Here's the drawing with two shaded views (mm, measured from the low corner). I have some questions. A direction names the side the tool comes from. Coordinates: 2 decimals unless noted, no trailing zeros. Loops run counter-clockwise (first coordinate to the right, second up) from the corner with the lowest first, then second, coordinate; pieces in that order, holes last. Notation, with made-up numbers: (86, 72) - (111, 72) arc R21 ccw to (111, 109) - close; hole circle Ø7 at (89, -12). An arc over 180 degrees is marked (long way). Use a Markdown table: item, result.
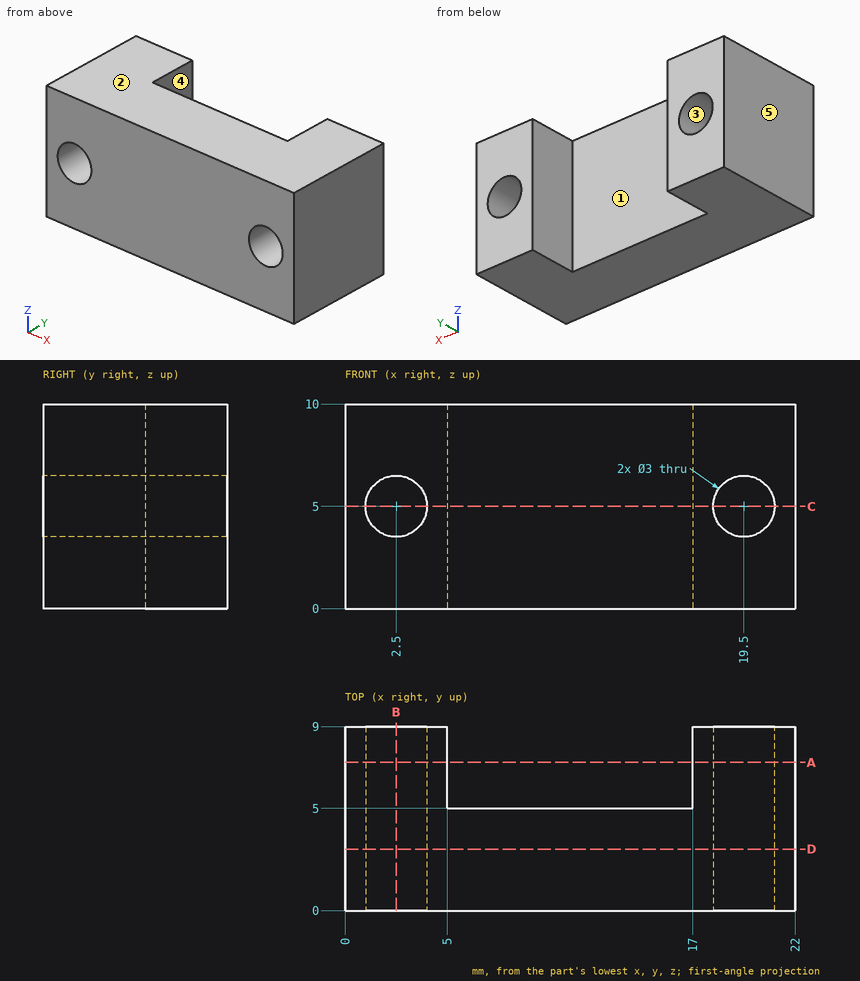
Q1. Please list where these lines run through material, in increasing order: L1, parallel to X at y = 2.5, z = 5; L2, parallel to Z at x = 19.5, y = 5; L3, parallel to X at y = 1.75, z = 6.25. Write a range as from..to.
Check values:
| item | result |
|---|---|
| L1 | 0..1, 4..18, 21..22 |
| L2 | 0..3.5, 6.5..10 |
| L3 | 0..1.67, 3.33..18.67, 20.33..22 |
Q2. If we mould it in two halves opening along Z, with no side actions, what happens to the marked faces 1, 2 and 3? For each: pulls with the +Z half, pulls with the -Z half, needs draft (parallel to the pull), parting line crosses it, or undercut.
Check values:
| item | result |
|---|---|
| face 1 | needs draft |
| face 2 | pulls with the +Z half |
| face 3 | undercut |
Q3. I want a section at D-D, the plane y = 3. Write out the boundary of the cut face in (x, z), then the cut area to 3 significant figures.
Check values:
| item | result |
|---|---|
| outline | (0, 0) - (22, 0) - (22, 10) - (0, 10) - close; hole circle Ø3 at (2.5, 5); hole circle Ø3 at (19.5, 5) |
| area | 206 mm^2 |
Q4. I want a section at A-A, the plane y = 7.25. Write out the boundary of the cut face in (x, z).
Check values:
| item | result |
|---|---|
| outline | (0, 0) - (5, 0) - (5, 10) - (0, 10) - close; (17, 0) - (22, 0) - (22, 10) - (17, 10) - close; hole circle Ø3 at (2.5, 5); hole circle Ø3 at (19.5, 5) |
Q5. Which directions (+Z, -Z, +X, -X, +Y, -Y) give clear straight access to the entire face, cutting with the end or side of a thin tool? Please do the marked faces 4 and 5.
Check values:
| item | result |
|---|---|
| face 4 | +Z, -Z, +Y |
| face 5 | +Z, -Z, -X, +Y, -Y |
Q6. Will these pins go through, and if not, where does the flat tip stop? P1, Ø2, axis at x = 10.5, y = 7.5, coming from the -Z side; P2, Ø3, axis at x = 10.5, z = 4, coming from the +Y side.
Check values:
| item | result |
|---|---|
| P1 | through |
| P2 | y = 5 |
Q7. I want a section at C-C, the plane z = 5. Write out the boundary of the cut face in (x, y).
Check values:
| item | result |
|---|---|
| outline | (0, 0) - (1, 0) - (1, 9) - (0, 9) - close; (4, 0) - (18, 0) - (18, 9) - (17, 9) - (17, 5) - (5, 5) - (5, 9) - (4, 9) - close; (21, 0) - (22, 0) - (22, 9) - (21, 9) - close |
Q8. I want a section at B-B, the plane x = 2.5. Write out the boundary of the cut face in (y, z), then the cut area to 3 significant figures.
Check values:
| item | result |
|---|---|
| outline | (0, 0) - (9, 0) - (9, 3.5) - (0, 3.5) - close; (0, 6.5) - (9, 6.5) - (9, 10) - (0, 10) - close |
| area | 63.0 mm^2 |
